The listing builds one solid part. Answer for the finished solid, in the listing's coordinates (mm). A direction names the side the tool comes from. Round coordinates to 2 decimals unless told otherwise and drop trailing zeros. Write each loop counter-clockwise with the first axis right and the second up, starting at its lowest first coordinate (ties: lowest second). Pieces come first, ordered by that corner, then holes.
(1) Each of these flat-tipped pins is pushed along its axis until it touches: pin 1 Ø3 at (y, z) = (-48, 4.5) entering from -X; pin 2 Ø2 at (y, z) = (-50.5, 6.5) entering from -X; pin 3 Ø0.6 at (x, z) = (-22, 0) entering from +Y; pin 4 Ø6 at (x, y) = (-12, -36) entering from +Z. Where does it stop, or does it pass through?
(2) A cutting plane is placed at D-D, the plane x = -13. Give the vertices of the cut face in (y, z).
(3) The mould has two halves that part along X. Classify faces 1 (the face through (25, -39, 2)), 2 (the face through (-26.5, -40, 2)), 3 (the face through (-8, -50, 8)): +X half, -X half, draft (parallel to the pull), parting line (faces both ways), or undercut.
(4) A cutting plane is placed at B-B, the plane y = -33.25. Give the vertices of the cut face in (x, z), and give its area (3 significant figures).
(5) A cutting plane is placed at C-C, the plane z = 2.5. Give the vertices of the cut face in (x, y).
(6) For faces 4 (the face through (-6.75, -50, 6)), 5 (the face through (0, -39, 0.5)), 6 (the face through (-19.25, -50, 6)), 7 (the face through (26.5, -40, 2)), 8 (the face through (-9.25, -50, 6)), determine the directions among +Z, -Z, +X, -X, +Y, -Y from which every point of the face is accessible in a straight line to the end or side of a thin tool.
(7) A cutting plane is placed at A-A, the plane z = 6.5. Give the vertices of the cut face in (x, y).
(8) Find the intervals of material crossed by probe 1 along X at (y, z) = (-30.25, 3.75); probe 2 along Z at (x, y) = (-5, -47.75); probe 3 along Y at (x, z) = (8, 2.25), in increasing order.
from build123d import *

# Parameters (mm, degrees)
SKETCH010_W     = 53
SKETCH010_H     = 22.5
PAD006_DEPTH    = 4
SKETCH011_W     = 50
SKETCH011_H     = 20
POCKET004_DEPTH = 3.5
SKETCH012_W     = 2.5
SKETCH012_H     = 2.5
PAD007_DEPTH    = 4
SKETCH016_W     = 3
SKETCH016_H     = 10
POCKET006_DEPTH = 0.501


with BuildPart() as part:
    # Sketch010 → Pad006 (new body)
    with BuildSketch(Plane.XY):
        Rectangle(SKETCH010_W, SKETCH010_H)
    extrude(amount=PAD006_DEPTH)

    # Sketch011 (on Face6 of Pad006) → Pocket004 (cut)
    with BuildSketch(Plane.XY.offset(4)):
        with Locations((0, 1.25)):
            Rectangle(SKETCH011_W, SKETCH011_H)
    extrude(amount=-POCKET004_DEPTH, mode=Mode.SUBTRACT)

    # Sketch012 (on Face4 of Pocket004) → Pad007 (join)
    with BuildSketch(Plane.XY.offset(4)):
        with Locations((-18, -10)):
            Rectangle(SKETCH012_W, SKETCH012_H)
        with Locations((-13, -10)):
            Rectangle(SKETCH012_W, SKETCH012_H)
        with Locations((-8, -10)):
            Rectangle(SKETCH012_W, SKETCH012_H)
    extrude(amount=PAD007_DEPTH)

    # Sketch016 (on Face6 of Pad007) → Pocket006 (cut, through all)
    with BuildSketch(Plane.XY.offset(0.5)):
        with Locations((-22.5, 6.25)):
            Rectangle(SKETCH016_W, SKETCH016_H)
    extrude(amount=-POCKET006_DEPTH, mode=Mode.SUBTRACT)


with BuildPart() as part_1:
    # Body003 placement: moved
    add(part.part.moved(Location((0, -40, 0))))


solid = part_1.part
Solutions:
1. pin 1: stops at x = -26.5
1. pin 2: stops at x = -19.25
1. pin 3: stops at y = -38.75
1. pin 4: stops at z = 0.5
2. outline: (-51.25, 0) - (-28.75, 0) - (-28.75, 0.5) - (-48.75, 0.5) - (-48.75, 8) - (-51.25, 8) - close
3. face 1: undercut
3. face 2: -X half
3. face 3: draft
4. outline: (-26.5, 0) - (-24, 0) - (-24, 0.5) - (-25, 0.5) - (-25, 4) - (-26.5, 4) - close; (-21, 0) - (26.5, 0) - (26.5, 4) - (25, 4) - (25, 0.5) - (-21, 0.5) - close
4. area: 35.5 mm2
5. outline: (-26.5, -51.25) - (26.5, -51.25) - (26.5, -28.75) - (25, -28.75) - (25, -48.75) - (-25, -48.75) - (-25, -28.75) - (-26.5, -28.75) - close
6. face 4: +Z, +X, +Y, -Y
6. face 5: +Z, +Y
6. face 6: +Z, -X, +Y, -Y
6. face 7: +Z, -Z, +X, +Y, -Y
6. face 8: +Z, +Y, -Y
7. outline: (-19.25, -51.25) - (-16.75, -51.25) - (-16.75, -48.75) - (-19.25, -48.75) - close; (-14.25, -51.25) - (-11.75, -51.25) - (-11.75, -48.75) - (-14.25, -48.75) - close; (-9.25, -51.25) - (-6.75, -51.25) - (-6.75, -48.75) - (-9.25, -48.75) - close
8. probe 1: x = -26.5 to -25, 25 to 26.5
8. probe 2: z = 0 to 0.5
8. probe 3: y = -51.25 to -48.75
